Work out the finished part from the listing and answer in its coordinate system (mm). Face numbers are marked on the shaded views. A direction names the side the tool comes from. Give positions to 0.01 mm unless a question says otherwise; leave off trailing zeros. Loops run counter-clockwise (first coordinate to the right, second up) from the corner with the lowest first, then second, coordinate; pieces in that order, holes last. Notation, with made-up numbers: (3.5, -21.5) - (60.5, -21.5) arc R7 ccw to (60.5, -10.5) - close; hole circle Ø1 at (-1, -17.5). An arc over 180 degrees is marked (long way). Use one line per item in the form item = value. Start each with the question number.
from build123d import *

# Parameters (mm, degrees)
F0_W     = 145
F0_H     = 82
F1_DEPTH = 200


with BuildPart() as f1:
    # F0 (on Right) → F1 (new body)
    with BuildSketch(Plane.YZ):
        with Locations((72.5, 41)):
            Rectangle(F0_W, F0_H)
        with BuildLine():
            Line((69, 78), (72.5, 78))
            Line((72.5, 78), (76, 78))
            Line((76, 78), (76, 79.3))
            Line((76, 79.3), (103, 79.3))
            Line((103, 79.3), (103, 78))
            Line((103, 78), (110, 78))
            Line((110, 78), (110, 79.3))
            Line((110, 79.3), (128, 79.3))
            Line((128, 79.3), (128, 78))
            Line((128, 78), (136.45, 78))
            Line((136.45, 78), (136.45, 77.6))
            ThreePointArc((136.45, 77.6), (137.6, 76.45), (138.75, 77.6))
            ThreePointArc((138.75, 77.6), (141.7374368671, 78.8374368671), (140.5, 75.85))
            ThreePointArc((140.5, 75.85), (139.35, 74.7), (140.5, 73.55))
            Line((140.5, 73.55), (142.6, 73.55))
            Line((142.6, 73.55), (142.6, 57))
            Line((142.6, 57), (140.0795047916, 57))
            Line((140.0795047916, 57), (140.0795047916, 55.5))
            Line((140.0795047916, 55.5), (142.6, 55.5))
            Line((142.6, 55.5), (142.6, 45.9740793705))
            Line((142.6, 45.9740793705), (141.8683309853, 45.9740793705))
            Line((141.8683309853, 45.9740793705), (142, 41))
            Line((142, 41), (141.8683309853, 36.0259206295))
            Line((141.8683309853, 36.0259206295), (142.6, 36.0259206295))
            Line((142.6, 36.0259206295), (142.6, 26.5))
            Line((142.6, 26.5), (140.0795047916, 26.5))
            Line((140.0795047916, 26.5), (140.0795047916, 25))
            Line((140.0795047916, 25), (142.6, 25))
            Line((142.6, 25), (142.6, 8.45))
            Line((142.6, 8.45), (140.5, 8.45))
            ThreePointArc((140.5, 8.45), (139.35, 7.3), (140.5, 6.15))
            ThreePointArc((140.5, 6.15), (141.7374368671, 3.1625631329), (138.75, 4.4))
            ThreePointArc((138.75, 4.4), (137.6, 5.55), (136.45, 4.4))
            Line((136.45, 4.4), (136.45, 4))
            Line((136.45, 4), (128, 4))
            Line((128, 4), (128, 2.7))
            Line((128, 2.7), (110, 2.7))
            Line((110, 2.7), (110, 4))
            Line((110, 4), (103, 4))
            Line((103, 4), (103, 2.7))
            Line((103, 2.7), (76, 2.7))
            Line((76, 2.7), (76, 4))
            Line((76, 4), (72.5, 4))
            Line((72.5, 4), (69, 4))
            Line((69, 4), (69, 2.7))
            Line((69, 2.7), (42, 2.7))
            Line((42, 2.7), (42, 4))
            Line((42, 4), (35, 4))
            Line((35, 4), (35, 2.7))
            Line((35, 2.7), (17, 2.7))
            Line((17, 2.7), (17, 4))
            Line((17, 4), (8.55, 4))
            Line((8.55, 4), (8.55, 4.4))
            ThreePointArc((8.55, 4.4), (7.4, 5.55), (6.25, 4.4))
            ThreePointArc((6.25, 4.4), (3.2625631329, 3.1625631329), (4.5, 6.15))
            ThreePointArc((4.5, 6.15), (5.65, 7.3), (4.5, 8.45))
            Line((4.5, 8.45), (2.4, 8.45))
            Line((2.4, 8.45), (2.4, 25))
            Line((2.4, 25), (4.9204952084, 25))
            Line((4.9204952084, 25), (4.9204952084, 26.5))
            Line((4.9204952084, 26.5), (2.4, 26.5))
            Line((2.4, 26.5), (2.4, 36.0259206295))
            Line((2.4, 36.0259206295), (3.1316690147, 36.0259206295))
            Line((3.1316690147, 36.0259206295), (3, 41))
            Line((3, 41), (3.1316690147, 45.9740793705))
            Line((3.1316690147, 45.9740793705), (2.4, 45.9740793705))
            Line((2.4, 45.9740793705), (2.4, 55.5))
            Line((2.4, 55.5), (4.9204952084, 55.5))
            Line((4.9204952084, 55.5), (4.9204952084, 57))
            Line((4.9204952084, 57), (2.4, 57))
            Line((2.4, 57), (2.4, 73.55))
            Line((2.4, 73.55), (4.5, 73.55))
            ThreePointArc((4.5, 73.55), (5.65, 74.7), (4.5, 75.85))
            ThreePointArc((4.5, 75.85), (3.2625631329, 78.8374368671), (6.25, 77.6))
            ThreePointArc((6.25, 77.6), (7.4, 76.45), (8.55, 77.6))
            Line((8.55, 77.6), (8.55, 78))
            Line((8.55, 78), (17, 78))
            Line((17, 78), (17, 79.3))
            Line((17, 79.3), (35, 79.3))
            Line((35, 79.3), (35, 78))
            Line((35, 78), (42, 78))
            Line((42, 78), (42, 79.3))
            Line((42, 79.3), (69, 79.3))
            Line((69, 79.3), (69, 78))
        make_face(mode=Mode.SUBTRACT)
    extrude(amount=F1_DEPTH)


solid = f1.part
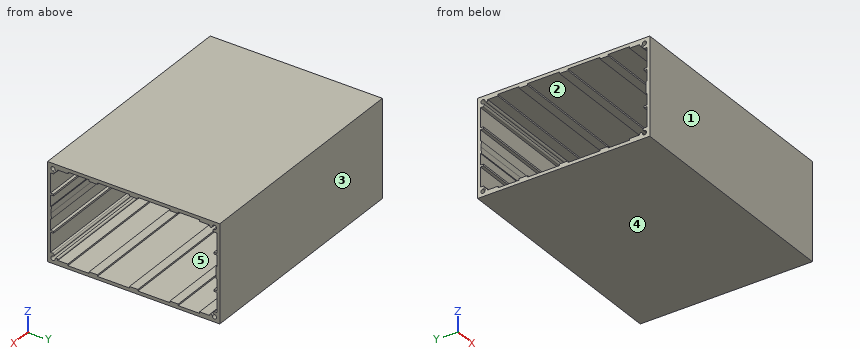
1) A cutting plane is placed at B-B (y = 94). Give the vertices of the cut face in (x, z), plus the area to 3 significant figures.
2) Find the intervals of material crossed by probe 1 along Z at (x, y) = (65, 4.5); probe 2 along Y at (x, z) = (52.5, 4.4); probe 3 along Y at (x, z) = (86.5, 42), in increasing order.
3) A tool of negligible diameter and unlimited length cuts with its end or side. For the marked faces 1 and 2, from which of +Z, -Z, +X, -X, +Y, -Y can it reach the whole face along a straight path? Write none if from no direction.
4) A flat-ended cylindrical pin translates along its axis: pin 1 Ø2 at (y, z) = (4.5, 4.4) entering from +X. Find the tip coordinate at first contact, or state that the pin passes through.
5) Determine the mould class of the marked faces 3, 4 and 5 for opening direction Y: released by +Y, released by -Y, zero draft, split by the parting line, or undercut.
6) A cutting plane is placed at A-A (z = 53). Give the vertices of the cut face in (x, y).
Answer sheet:
q1.outline = (0, 0) - (200, 0) - (200, 2.7) - (0, 2.7) - close; (0, 79.3) - (200, 79.3) - (200, 82) - (0, 82) - close
q1.area = 1,080 mm²
q2.probe_1 = 0 to 2.65, 6.15 to 8.45, 25 to 26.5, 55.5 to 57, 73.55 to 75.85, 79.35 to 82
q2.probe_2 = 0 to 2.75, 6.25 to 8.55, 136.45 to 138.75, 142.25 to 145
q2.probe_3 = 0 to 3.03, 141.97 to 145
q3.face_1 = +Z, -Z, +X, -X, -Y
q3.face_2 = +X, -X
q4.pin_1 = through
q5.face_3 = released by +Y
q5.face_4 = zero draft
q5.face_5 = undercut
q6.outline = (0, 0) - (200, 0) - (200, 2.4) - (0, 2.4) - close; (0, 142.6) - (200, 142.6) - (200, 145) - (0, 145) - close
